```python
from build123d import *
from OCP.BRepFilletAPI import BRepFilletAPI_MakeFillet

# Parameters (mm, degrees)
SKETCH1_W               = 55.36
SKETCH1_H               = 30.8
BOSS_EXTRUDE1_DEPTH     = 2
SKETCH3_W               = 2
SKETCH3_H               = 5
BOSS_EXTRUDE3_DEPTH     = 16.85
SKETCH5_W               = 16
SKETCH5_H               = 20
CUT_EXTRUDE1_DEPTH      = 37.860071894
FILLET1_R1              = 6
FILLET1_R2              = 4
FILLET2_R               = 1.5
BOSS_EXTRUDE4_START     = -3
BOSS_EXTRUDE4_DEPTH     = 17
CHAMFER1_SIZE           = 0.97411139
CHAMFER1_SIZE_2         = 1.5
FILLET6_R               = 0.5
FILLET7_R               = 4
CUT_EXTRUDE2_DEPTH      = 8
CUT_EXTRUDE2_DEPTH_BACK = 5
FILLET8_START           = -27.68
FILLET8_DEPTH           = 2
FILLET8_START_2         = 12.8999999
FILLET8_2_DEPTH         = 2.5000001
FILLET8_START_3         = -8.4
FILLET8_3_DEPTH         = 3.0000001
FILLET8_START_4         = -25.68
FILLET8_4_DEPTH         = 14.5


with BuildPart() as part:
    # Sketch1 → Boss-Extrude1 (new body)
    with BuildSketch(Plane(origin=(0, 0, 0), x_dir=(1, 0, 0), z_dir=(0, 1, 0))):
        Rectangle(SKETCH1_W, SKETCH1_H)
    extrude(amount=BOSS_EXTRUDE1_DEPTH)

    # Sketch3 → Boss-Extrude3 (add)
    with BuildSketch(Plane(origin=(0, 2, 0), x_dir=(1, 0, 0), z_dir=(0, 1, 0))):
        with Locations((-26.68, 10.9)):
            Rectangle(SKETCH3_W, SKETCH3_H)
        Polygon((-27.68, 15.4), (-27.68, 13.4), (-25.68, 13.4), (25.68, 13.4), (25.68, -13.4), (-11.18, -13.4), (-11.18, -15.4), (27.68, -15.4), (27.68, 15.4), align=None)
    extrude(amount=BOSS_EXTRUDE3_DEPTH)

    # Sketch5 → Cut-Extrude1 (cut, through all)
    with BuildSketch(Plane(origin=(0, 0, 0), x_dir=(0, 0, -1), z_dir=(1, 0, 0))):
        with Locations((0, 14)):
            Rectangle(SKETCH5_W, SKETCH5_H)
    extrude(amount=CUT_EXTRUDE1_DEPTH, mode=Mode.SUBTRACT)

    # Fillet1: one fillet with a radius per group of edges: ONE call of the kernel's fillet builder (fillet() takes one radius for all edges)
    fillet1_edges_1 = [part.edges().sort_by_distance(p)[0] for p in [
        (27.68, 9.425, -15.4),
        (27.68, 9.425, 15.4),
        (-27.68, 9.425, -15.4),
        (-27.68, 1, 15.4),
    ]]
    fillet1_edges_2 = [part.edges().sort_by_distance(p)[0] for p in [
        (25.68, 10.425, -13.4),
        (25.68, 10.425, 13.4),
        (-25.68, 10.425, -13.4),
    ]]
    fillet1 = BRepFilletAPI_MakeFillet(part.part.solid().wrapped)
    for e in fillet1_edges_1:
        fillet1.Add(FILLET1_R1, e.wrapped)
    for e in fillet1_edges_2:
        fillet1.Add(FILLET1_R2, e.wrapped)
    add(Compound.cast(fillet1.Shape()), mode=Mode.REPLACE)

    # Fillet2
    fillet2_edges = [part.edges().sort_by_distance(p)[0] for p in [
        (0, 0, 15.4),
        (27.68, 0, 0),
        (-27.68, 0, 0),
        (0, 0, -15.4),
        (25.922640687, 0, -13.642640687),
        (25.922640687, 0, 13.642640687),
        (-25.922640687, 0, -13.642640687),
        (-25.922640687, 0, 13.642640687),
    ]]
    fillet(fillet2_edges, radius=FILLET2_R)

    # Sketch4 → Boss-Extrude4 (add)
    with BuildSketch(Plane.ZY.offset(10.18).offset(BOSS_EXTRUDE4_START)):
        Polygon((-13.4, 18.85), (-11.971851993, 17.85), (-13.4, 16.85), align=None)
        Polygon((13.4, 18.85), (11.971851993, 17.85), (13.4, 16.85), align=None)
    extrude(amount=-BOSS_EXTRUDE4_DEPTH)

    # Chamfer1
    # the kernel refuses this chamfer: 1.5, 0.97411139 mm, written as the material it adds along each edge
    with BuildSketch(Plane(origin=(9.82, 12.9733385, 13.4), x_dir=(1, 0, 0), z_dir=(0, 1, 0))) as chamfer1_piece_1_section:
        Polygon((CHAMFER1_SIZE, 0), (0, CHAMFER1_SIZE_2), (0, 0), align=None)
    chamfer1_piece_1 = extrude(amount=5.8766615, mode=Mode.PRIVATE)
    chamfer1_piece_1 = split(chamfer1_piece_1, bisect_by=Plane(origin=(9.82, 15.574617411, 15.221435103), z_dir=(0, 0.8191520442889897, 0.5735764363510492)), keep=Keep.TOP, mode=Mode.PRIVATE)
    chamfer1_piece_1 = split(chamfer1_piece_1, bisect_by=Plane(origin=(9.82, 16.916637554, 10.638872277), z_dir=(0, -0.8191520442889973, 0.5735764363510382)), keep=Keep.TOP, mode=Mode.PRIVATE)
    add(chamfer1_piece_1)
    with BuildSketch(Plane(origin=(-7.18, 12.9733385, 13.4), x_dir=(-1, 0, 0), z_dir=(0, 1, 0))) as chamfer1_piece_2_section:
        Polygon((CHAMFER1_SIZE, 0), (0, -CHAMFER1_SIZE_2), (0, 0), align=None)
    chamfer1_piece_2 = extrude(amount=5.8766615, mode=Mode.PRIVATE)
    chamfer1_piece_2 = split(chamfer1_piece_2, bisect_by=Plane(origin=(-7.18, 15.574617411, 15.221435103), z_dir=(0, 0.8191520442889897, 0.5735764363510492)), keep=Keep.TOP, mode=Mode.PRIVATE)
    chamfer1_piece_2 = split(chamfer1_piece_2, bisect_by=Plane(origin=(-7.18, 16.916637554, 10.638872277), z_dir=(0, -0.8191520442889973, 0.5735764363510382)), keep=Keep.TOP, mode=Mode.PRIVATE)
    add(chamfer1_piece_2)
    with BuildSketch(Plane(origin=(9.82, 12.9733385, -13.4), x_dir=(1, 0, 0), z_dir=(0, 1, 0))) as chamfer1_piece_3_section:
        Polygon((CHAMFER1_SIZE, 0), (0, -CHAMFER1_SIZE_2), (0, 0), align=None)
    chamfer1_piece_3 = extrude(amount=5.8766615, mode=Mode.PRIVATE)
    chamfer1_piece_3 = split(chamfer1_piece_3, bisect_by=Plane(origin=(9.82, 15.574617411, -15.221435103), z_dir=(0, 0.8191520442889897, -0.5735764363510492)), keep=Keep.TOP, mode=Mode.PRIVATE)
    chamfer1_piece_3 = split(chamfer1_piece_3, bisect_by=Plane(origin=(9.82, 16.916637554, -10.638872277), z_dir=(0, -0.8191520442889973, -0.5735764363510382)), keep=Keep.TOP, mode=Mode.PRIVATE)
    add(chamfer1_piece_3)
    with BuildSketch(Plane(origin=(-7.18, 12.9733385, -13.4), x_dir=(-1, 0, 0), z_dir=(0, 1, 0))) as chamfer1_piece_4_section:
        Polygon((CHAMFER1_SIZE, 0), (0, CHAMFER1_SIZE_2), (0, 0), align=None)
    chamfer1_piece_4 = extrude(amount=5.8766615, mode=Mode.PRIVATE)
    chamfer1_piece_4 = split(chamfer1_piece_4, bisect_by=Plane(origin=(-7.18, 15.574617411, -15.221435103), z_dir=(0, 0.8191520442889897, -0.5735764363510492)), keep=Keep.TOP, mode=Mode.PRIVATE)
    chamfer1_piece_4 = split(chamfer1_piece_4, bisect_by=Plane(origin=(-7.18, 16.916637554, -10.638872277), z_dir=(0, -0.8191520442889973, -0.5735764363510382)), keep=Keep.TOP, mode=Mode.PRIVATE)
    add(chamfer1_piece_4)

    # Fillet6
    fillet6_edges = [part.edges().sort_by_distance(p)[0] for p in [
        (-25.68, 2, -8.9),
        (5.25, 2, 13.4),
        (0, 2, -13.4),
        (25.68, 2, 0),
        (24.508427125, 2, -12.228427125),
        (24.508427125, 2, 12.228427125),
        (-24.508427125, 2, -12.228427125),
    ]]
    fillet(fillet6_edges, radius=FILLET6_R)

    # Fillet7
    fillet7_edges = [part.edges().sort_by_distance(p)[0] for p in [
        (26.68, 4, -8),
        (26.68, 4, 8),
    ]]
    fillet(fillet7_edges, radius=FILLET7_R)

    # Sketch6 → Cut-Extrude2 (cut, two sides: drawn at the far end of the back side and taken through both)
    with BuildSketch(Plane(origin=(0, 0, 0), x_dir=(0, 0, -1), z_dir=(1, 0, 0)).offset(-CUT_EXTRUDE2_DEPTH_BACK)):
        Polygon((-15.025755833, 18.85), (-14.4, 17.97951196), (-13.841478047, 18.85), align=None)
        Polygon((13.841478047, 18.85), (15.025755833, 18.85), (14.4, 17.97951196), align=None)
    extrude(amount=CUT_EXTRUDE2_DEPTH + CUT_EXTRUDE2_DEPTH_BACK, mode=Mode.SUBTRACT)

    # Fillet8: read off the stored shape, not the designer's step
    # Fillet8 outline → Fillet8 (add)
    with BuildSketch(Plane.YZ.offset(FILLET8_START)):
        with BuildLine():
            Line((2, -8.4), (5, -8.4))
            ThreePointArc((5, -8.4), (2.878679656, -7.521320344), (2, -5.4))
            Line((2, -5.4), (2, -8.4))
        make_face()
    extrude(amount=FILLET8_DEPTH)

    # Fillet8 2 outline → Fillet8 2 (add)
    with BuildSketch(Plane.XY.offset(FILLET8_START_2)):
        with BuildLine():
            ThreePointArc((-11.18, 5), (-12.058679656, 2.878679656), (-14.18, 2))
            Line((-14.18, 2), (-11.18, 2))
            Line((-11.18, 2), (-11.18, 5))
        make_face()
    extrude(amount=FILLET8_2_DEPTH)

    # Fillet8 3 outline → Fillet8 3 (add)
    with BuildSketch(Plane.XY.offset(FILLET8_START_3)):
        with BuildLine():
            ThreePointArc((-25.18, 2), (-25.533553391, 2.146446609), (-25.68, 2.5))
            Line((-25.68, 2.5), (-25.68, 2))
            Line((-25.68, 2), (-25.18, 2))
        make_face()
    extrude(amount=FILLET8_3_DEPTH)

    # Fillet8 4 outline → Fillet8 4 (cut)
    with BuildSketch(Plane.YZ.offset(FILLET8_START_4)):
        with BuildLine():
            ThreePointArc((2.5, 13.4), (2.146446609, 13.253553391), (2, 12.9))
            Line((2, 12.9), (5, 12.8999999))
            Line((5, 12.8999999), (5, 13.4))
            Line((5, 13.4), (2.5, 13.4))
        make_face()
        with BuildLine():
            ThreePointArc((2, -5.4), (2.127718677, -6.266025404), (2.5, -7.058312396))
            Line((2.5, -7.058312396), (2.5, -5.3999999))
            Line((2.5, -5.3999999), (2, -5.4))
        make_face()
    extrude(amount=FILLET8_4_DEPTH, mode=Mode.SUBTRACT)


solid = part.part
```
For this review, take the finished solid that the model builds, in its own axes (mm). A direction names the side the tool comes from. Round coordinates to 2 decimals unless told otherwise and drop trailing zeros. Write each loop counter-clockwise with the first axis right and the second up, starting at its lowest first coordinate (ties: lowest second). Pieces come first, ordered by that corner, then holes. Notation, with made-up numbers: (23, 44) -> (82, 44) arc R32 cw to (82, 70) -> close; hole circle Ø10 at (-8, 0.5). An arc over 180 degrees is marked (long way). One line per question, with ' | ' between items. Start each with the question number.
(1) Add section D-D, the plane x = -21. Write out the cut boundary in (y, z).
(2) Insertion check: P1, Ø2, axis at y = 10, z = 14.5, coming from the -X side; P2, Ø2, axis at x = 27, y = 15, coming from the +Z side; P3, Ø0.6, axis at x = 27, y = 15, coming from the -Z side. Each pin has a flat end and moves straight along its axis. Give the tip position at first contact, or say it passes through.
(3) Tool access review of faces 4 (the face through (-7.8, 17.836, -12.855)), 5 (the face through (0, 11, -13.4)), 6 (the face through (27, 13, 8)), 7 (the face through (-27, 12, -8.4)): name each direction out of +Z, -Z, +X, -X, +Y, -Y from which nothing blocks a thin tool from reaching the whole face with its end or side.
(4) For line 1 along Z through (x, y) = (16, 5.5); line 2 along Y through (x, z) = (23.5, -5); line 3 along X through (y, z) = (9.5, 9), list the stretches that pass through material, from the lowest coordinate up. Write a range as from..to.
(5) Add section B-B, the plane x = -3. Write out the cut boundary in (y, z).
(6) Mouldability with a two-part tool opening along Z and no side actions: class faces 1 (the face through (-27.2, 0.4, 0.1)), 2 (the face through (-25.969, 10.054, -13.596)), 3 (the face through (26.694, 5.141, -6.797)) as released by +Z, released by -Z, zero draft, split by the parting line, or undercut.
(7) Add section C-C, the plane z = 2.5. Write out the cut boundary in (x, y).
(8) Add section A-A, the plane y = 15.5. Write out the cut boundary in (x, z).
Answer list:
1) outline: (0, -13.9) arc R1.5 ccw to (1.5, -15.4) -> (18.85, -15.4) -> (18.85, -13.4) -> (2.5, -13.4) arc R0.5 cw to (2, -12.9) -> (2, 15.4) -> (1.5, 15.4) arc R1.5 ccw to (0, 13.9) -> close
2) P1: x = -11.18 | P2: z = 13.56 | P3: z = -12.69
3) face 4: +Y | face 5: none | face 6: +X, -X, +Y | face 7: +Z, -X, +Y
4) line 1: -15.4..-13.4, 13.4..15.4 | line 2: 0..2 | line 3: 25.68..27.68
5) outline: (0, -13.9) arc R1.5 ccw to (1.5, -15.4) -> (18.85, -15.4) -> (18.85, -15.03) -> (17.98, -14.4) -> (18.85, -13.84) -> (18.85, -13.4) -> (17.85, -11.97) -> (16.85, -13.4) -> (2.5, -13.4) arc R0.5 cw to (2, -12.9) -> (2, 12.9) arc R0.5 cw to (2.5, 13.4) -> (16.85, 13.4) -> (17.85, 11.97) -> (18.85, 13.4) -> (18.85, 13.84) -> (17.98, 14.4) -> (18.85, 15.03) -> (18.85, 15.4) -> (1.5, 15.4) arc R1.5 ccw to (0, 13.9) -> close
6) face 1: zero draft | face 2: released by -Z | face 3: undercut
7) outline: (-27.68, 1.5) arc R1.5 ccw to (-26.18, 0) -> (26.18, 0) arc R1.5 ccw to (27.68, 1.5) -> (27.68, 4) -> (25.68, 4) -> (25.68, 2.5) arc R0.5 cw to (25.18, 2) -> (-27.68, 2) -> close
8) outline: (-27.68, -9.4) arc R6 ccw to (-21.68, -15.4) -> (21.68, -15.4) arc R6 ccw to (27.68, -9.4) -> (27.68, -8) -> (25.68, -8) -> (25.68, -9.4) arc R4 cw to (21.68, -13.4) -> (-21.68, -13.4) arc R4 cw to (-25.68, -9.4) -> (-25.68, -8.4) -> (-27.68, -8.4) -> close; (-11.18, 13.4) -> (21.68, 13.4) arc R4 cw to (25.68, 9.4) -> (25.68, 8) -> (27.68, 8) -> (27.68, 9.4) arc R6 ccw to (21.68, 15.4) -> (-11.18, 15.4) -> close
